Verification items for the finished model (mm, model axes). A direction names the side the tool comes from. Coordinates: 2 decimals unless noted, no trailing zeros. Order: outer loops, then holes, each group sorted by start corner. A loop starts at its lowest first (then second) coordinate and runs counter-clockwise, first axis right, second up. Notation, with made-up numbers: (-26, 8.5) - (23, 8.5) arc R31 ccw to (23, 41.5) - close; hole circle Ø3 at (-40, -28). An arc over 180 degrees is marked (long way). Answer as CSV lines item,"result". Start each with the question number.
1. Section check C-C (y = -48). Record the cut outline in (x, z), and give its area (3 significant figures).
2. Material ranges on L1, parallel to Y at x = 71, z = 29; L2, parallel to Y at x = 67, z = 93.5; L3, parallel to X at y = -26.5, z = 85, recorded low to high. Write a range as [from, to].
3. Set-up check for faces 4 (the flat face through (12, -30, 94)), 5 (the flat face through (55, -22, 100)), 6 (the flat face through (8.24, -21.79, 49.3)): record each of +Z, -Z, +X, -X, +Y, -Y from which the full face is reachable in a straight line by a thin tool's end or side.
4. Mould release check, pull along X, two halves, no side actions. Record for faces 1 (the flat face through (5.91, -21.75, 49.3)), 2 (the flat face through (63.5, 19.2, 100)), 3 (the flat face through (31, 19.012, 49)): pulls with the +X half, pulls with the -X half, needs draft (parallel to the pull), parting line crosses it, or undercut.
5. Section check A-A (z = 72). Record the cut outline in (x, y), and give its area (3 significant figures).
6. Go/stop test with flat-tipped pins: pin 1 (2 mm diameter, centred on y = 20, z = 97, fed in from -X); pin 2 (1.9 mm diameter, centred on x = 51, y = -30.5, fed in from +Z); pin 3 (12 mm diameter, centred on y = -47, z = 79.5, fed in from -X). Record where each tip stops, or that it passes through.
7. Section check B-B (x = -5.5). Record the cut outline in (y, z), and give its area (3 significant figures).
from build123d import *

# Parameters (mm, degrees)
F1_DEPTH = 100
F2_W     = 4.05
F2_H     = 2
F3_DEPTH = 6


with BuildPart() as f1:
    # F0 (on Top) → F1 (new body)
    with BuildSketch(Plane.XY):
        with BuildLine():
            Line((76.0228561422, 21.0123993456), (-13.5848390123, 21.0123993456))
            ThreePointArc((-13.5848390123, 21.0123993456), (-16.1829152237, 19.5123993456), (-16.1829152237, 16.5123993456))
            Line((-16.1829152237, 16.5123993456), (28.6209323536, -61.0901410328))
            ThreePointArc((28.6209323536, -61.0901410328), (31.2190085649, -62.5901410328), (33.8170847763, -61.0901410328))
            Line((33.8170847763, -61.0901410328), (78.6209323536, 16.5123993456))
            ThreePointArc((78.6209323536, 16.5123993456), (78.6209323536, 19.5123993456), (76.0228561422, 21.0123993456))
        make_face()
        with BuildLine():
            ThreePointArc((-12.7188136086, 14.5123993456), (-12.7188136086, 17.5123993456), (-10.1207373972, 19.0123993456))
            Line((-10.1207373972, 19.0123993456), (72.5587545271, 19.0123993456))
            ThreePointArc((72.5587545271, 19.0123993456), (75.1568307385, 17.5123993456), (75.1568307385, 14.5123993456))
            Line((75.1568307385, 14.5123993456), (33.8170847763, -57.0901410328))
            ThreePointArc((33.8170847763, -57.0901410328), (31.2190085649, -58.5901410328), (28.6209323536, -57.0901410328))
            Line((28.6209323536, -57.0901410328), (-12.7188136086, 14.5123993456))
        make_face(mode=Mode.SUBTRACT)
    extrude(amount=F1_DEPTH)

    # F2 (on face) → F3 (cut)
    with BuildSketch(Plane.XY.offset(100)):
        with Locations((21.6940085649, 20.0123993456)):
            Rectangle(F2_W, F2_H)
        with Locations((40.7440085649, 20.0123993456)):
            Rectangle(F2_W, F2_H)
        Polygon((2.1760593725, -11.2862774299), (0.4440085649, -12.2862774299), (2.4690085649, -15.7936803152), (4.2010593725, -14.7936803152), align=None)
        Polygon((11.7010593725, -27.784061372), (9.9690085649, -28.784061372), (11.9940085649, -32.2914642573), (13.7260593725, -31.2914642573), align=None)
        Polygon((61.9940085649, -12.2862774299), (60.2619577574, -11.2862774299), (58.2369577574, -14.7936803152), (59.9690085649, -15.7936803152), align=None)
        Polygon((52.4690085649, -28.784061372), (50.7369577574, -27.784061372), (48.7119577574, -31.2914642573), (50.4440085649, -32.2914642573), align=None)
    extrude(amount=-F3_DEPTH, mode=Mode.SUBTRACT)


solid = f1.part
Evaluation:
1,outline,"(21.06, 0) - (23.37, 0) - (23.37, 100) - (21.06, 100) - close; (39.07, 0) - (41.37, 0) - (41.37, 100) - (39.07, 100) - close"
1,area,"462 mm²"
2,L1,"y = [3.31, 7.31], [19.01, 21.01]"
2,L2,"y = [-3.62, 0.38], [19.01, 21.01]"
2,L3,"x = [8.65, 10.96], [51.48, 53.79]"
3,face 4,"+Z"
3,face 5,"+Z, +X, -X, +Y, -Y"
3,face 6,"+Z, -Z"
4,face 1,"pulls with the -X half"
4,face 2,"needs draft"
4,face 3,"undercut"
5,outline,"(-16.18, 16.51) - (28.62, -61.09) arc R3 ccw to (33.82, -61.09) - (78.62, 16.51) arc R3 ccw to (76.02, 21.01) - (-13.58, 21.01) arc R3 ccw to start; hole (-12.72, 14.51) - (28.62, -57.09) arc R3 ccw to (33.82, -57.09) - (75.16, 14.51) arc R3 ccw to (72.56, 19.01) - (-10.12, 19.01) arc R3 ccw to start"
5,area,"579 mm²"
6,pin 1,"stops at x = -16.42"
6,pin 2,"stops at z = 94"
6,pin 3,"stops at x = 17.02"
7,outline,"(-1.99, 0) - (2.01, 0) - (2.01, 100) - (-1.99, 100) - close; (19.01, 0) - (21.01, 0) - (21.01, 100) - (19.01, 100) - close"
7,area,"600 mm²"
